Can you work these out from the model? Positions are in its coordinate system, mm. Face numbers are marked on the shaded views. A direction names the side the tool comes from. Give positions to 0.01 mm unless a question says otherwise; leave off trailing zeros. Loops run counter-clockwise (first coordinate to the right, second up) from the corner with the lowest first, then second, coordinate; pieces in that order, holes last.
from build123d import *

# Parameters (mm, degrees)
SKETCH1_R           = 19.05
SKETCH1_R_2         = 16.764
BOSS_EXTRUDE1_DEPTH = 31.75
BOSS_EXTRUDE2_START = -10.16
SKETCH2_R           = 16.764
SKETCH2_R_2         = 12.7
BOSS_EXTRUDE2_DEPTH = 20.32
CUT_EXTRUDE1_DEPTH  = 10.16


with BuildPart() as part:
    # Sketch1 → Boss-Extrude1 (new body)
    with BuildSketch(Plane.XY):
        Circle(SKETCH1_R)
        Circle(SKETCH1_R_2, mode=Mode.SUBTRACT)
    extrude(amount=-BOSS_EXTRUDE1_DEPTH)

    # Sketch2 → Boss-Extrude2 (add)
    with BuildSketch(Plane.XY.offset(BOSS_EXTRUDE2_START)):
        Circle(SKETCH2_R)
        Circle(SKETCH2_R_2, mode=Mode.SUBTRACT)
    extrude(amount=-BOSS_EXTRUDE2_DEPTH)

    # Sketch4 → Cut-Extrude1 (cut)
    with BuildSketch(Plane.XY):
        with BuildLine():
            Line((-7.290119387, 17.599905094), (-6.41530506, 15.487916483))
            ThreePointArc((-6.41530506, 15.487916483), (0, 16.764), (6.41530506, 15.487916483))
            Line((6.41530506, 15.487916483), (7.290119387, 17.599905094))
            ThreePointArc((7.290119387, 17.599905094), (0, 19.05), (-7.290119387, 17.599905094))
        make_face()
        with BuildLine():
            Line((17.599905094, -7.290119387), (15.487916483, -6.41530506))
            ThreePointArc((15.487916483, -6.41530506), (16.764, 0), (15.487916483, 6.41530506))
            Line((15.487916483, 6.41530506), (17.599905094, 7.290119387))
            ThreePointArc((17.599905094, 7.290119387), (19.05, 0), (17.599905094, -7.290119387))
        make_face()
        with BuildLine():
            Line((-7.290119387, -17.599905094), (-6.41530506, -15.487916483))
            ThreePointArc((-6.41530506, -15.487916483), (0, -16.764), (6.41530506, -15.487916483))
            Line((6.41530506, -15.487916483), (7.290119387, -17.599905094))
            ThreePointArc((7.290119387, -17.599905094), (0, -19.05), (-7.290119387, -17.599905094))
        make_face()
        with BuildLine():
            Line((-17.599905094, 7.290119387), (-15.487916483, 6.41530506))
            ThreePointArc((-15.487916483, 6.41530506), (-16.764, 0), (-15.487916483, -6.41530506))
            Line((-15.487916483, -6.41530506), (-17.599905094, -7.290119387))
            ThreePointArc((-17.599905094, -7.290119387), (-19.05, 0), (-17.599905094, 7.290119387))
        make_face()
    extrude(amount=-CUT_EXTRUDE1_DEPTH, mode=Mode.SUBTRACT)


solid = part.part
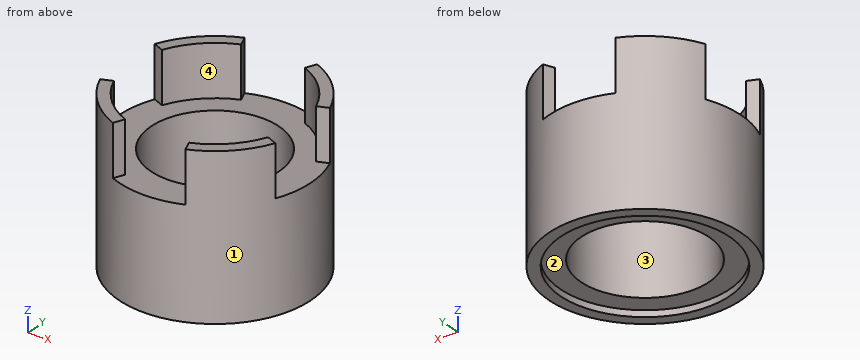
(1) Thinking about a two-plate mould opening in Y: for the marked faces 1 and 2, which applies, pulls with the +Y half, pulls with the -Y half, needs draft (parallel to the pull), parting line crosses it, or undercut?
Returned:
face 1: parting line crosses it
face 2: undercut
(2) Suppose I cut it at B-B on z = -2.5. List the corners of the cut face in (x, y) for me.
Returned:
outline: (-17.6, -7.29) arc R19.05 ccw to (-7.29, -17.6) - (-6.42, -15.49) arc R16.76 cw to (-15.49, -6.42) - close; (-17.6, 7.29) - (-15.49, 6.42) arc R16.76 cw to (-6.42, 15.49) - (-7.29, 17.6) arc R19.05 ccw to start; (6.42, -15.49) - (7.29, -17.6) arc R19.05 ccw to (17.6, -7.29) - (15.49, -6.42) arc R16.76 cw to start; (6.42, 15.49) arc R16.76 cw to (15.49, 6.42) - (17.6, 7.29) arc R19.05 ccw to (7.29, 17.6) - close
(3) Suppose I cut it at A-A on y = 0. List the corners of the cut face in (x, z) for me.
Returned:
outline: (-19.05, -31.75) - (-16.76, -31.75) - (-16.76, -30.48) - (-12.7, -30.48) - (-12.7, -10.16) - (-19.05, -10.16) - close; (12.7, -30.48) - (16.76, -30.48) - (16.76, -31.75) - (19.05, -31.75) - (19.05, -10.16) - (12.7, -10.16) - close
(4) Will these pins go through, and if not, where does the flat tip stop? P1, Ø1, axis at y = -14.5, z = -13, coming from the -X side; P2, Ø8, axis at x = 10.5, y = -7, coming from the -Z side; P3, Ø12, axis at x = -11.5, z = -12, coming from the -Y side.
Returned:
P1: stops at x = -12.92
P2: stops at z = -30.48
P3: stops at y = -18.24
(5) Suppose I cut it at D-D on y = 16. List the corners of the cut face in (x, z) for me, plus the area to 3 significant figures.
Returned:
outline: (-10.34, -31.75) - (-5, -31.75) - (-5, -30.48) - (5, -30.48) - (5, -31.75) - (10.34, -31.75) - (10.34, 0) - (6.63, 0) - (6.63, -10.16) - (-6.63, -10.16) - (-6.63, 0) - (-10.34, 0) - close
area: 509 mm2
(6) Which directions (+Z, -Z, +X, -X, +Y, -Y) give clear straight access to the entire face, cutting with the end or side of a thin tool? Please do the marked faces 3 and 4.
Returned:
face 3: +Z, -Z
face 4: +Z
(7) Please list where these lines run through material, in increasing order: probe 1 along Y at (x, z) = (0, -31); probe 2 along Y at (x, z) = (0, -21.25); probe 3 along X at (y, z) = (0.5, -20).
Returned:
probe 1: y = -19.05 to -16.76, 16.76 to 19.05
probe 2: y = -19.05 to -12.7, 12.7 to 19.05
probe 3: x = -19.04 to -12.69, 12.69 to 19.04
